from build123d import *

# Parameters (mm, degrees)
SKETCH006_R           = 114.3
PAD003_DEPTH          = 20
SKETCH007_R           = 4.25
HOLE001_DEPTH         = 75
HOLE001_TIPS_R        = 4.25
SKETCH008_R           = 4.25
HOLE002_DEPTH         = 200
POLARPATTERN001_COUNT = 3
POLARPATTERN001_ANGLE = 240


with BuildPart() as part:
    # Sketch006 → Pad003 (new body)
    with BuildSketch(Plane.XY):
        with BuildLine():
            ThreePointArc((50, -124.645457), (0, 134.3), (-50, -124.645457))
            Line((-50, -124.645457), (-50, -154.645457))
            Line((-50, -154.645457), (50, -154.645457))
            Line((50, -154.645457), (50, -124.645457))
        make_face()
        Circle(SKETCH006_R, mode=Mode.SUBTRACT)
    extrude(amount=PAD003_DEPTH)

    # Sketch007 (on Face3 of Pad003) → Hole001 (cut)
    with BuildSketch(Plane.XZ.offset(154.645457)):
        with Locations((-25, 10)):
            Circle(SKETCH007_R)
        with Locations((25, 10)):
            Circle(SKETCH007_R)
    extrude(amount=-HOLE001_DEPTH, mode=Mode.SUBTRACT)

    # Hole001 tips → Hole001 tip 1 section 0
    with BuildSketch(Plane.XZ.offset(79.645457), mode=Mode.PRIVATE) as hole001_tip_1_s0:
        with Locations((-25, 10)):
            Circle(HOLE001_TIPS_R)
    loft([hole001_tip_1_s0.sketch, Vertex(-25, -77.0918, 10)], mode=Mode.SUBTRACT)

    # Hole001 tips → Hole001 tip 2 section 0
    with BuildSketch(Plane.XZ.offset(79.645457), mode=Mode.PRIVATE) as hole001_tip_2_s0:
        with Locations((25, 10)):
            Circle(HOLE001_TIPS_R)
    loft([hole001_tip_2_s0.sketch, Vertex(25, -77.0918, 10)], mode=Mode.SUBTRACT)

    # Sketch008 → Hole002 (cut)
    with BuildSketch(Plane.XZ):
        with Locations((0, 10)):
            Circle(SKETCH008_R)
    hole002 = extrude(amount=-HOLE002_DEPTH, mode=Mode.SUBTRACT)

    # PolarPattern001: Hole002 ×3 about axis
    polarpattern001_axis = Axis((0, 0, 0), (0, 0, 1))
    for i in range(1, POLARPATTERN001_COUNT):
        add(hole002.rotate(polarpattern001_axis, i * POLARPATTERN001_ANGLE / (POLARPATTERN001_COUNT - 1)), mode=Mode.SUBTRACT)


solid = part.part
Input: part model. Units: mm. Frame: model coordinates. A direction names the side the tool comes from. Give positions to 0.01 mm unless a question says otherwise; leave off trailing zeros. Order: outer loops, then holes, each group sorted by start corner. A loop starts at its lowest first (then second) coordinate and runs counter-clockwise, first axis right, second up. Notation, with made-up numbers: (30.25, 75.5) - (84.25, 75.5) arc R38 ccw to (84.25, 113.5) - close; hole circle Ø2 at (74, 42.25). An arc over 180 degrees is marked (long way). Answer as a JSON object with one key per item and string values. Group by question number.
Q1. First-contact query: pin 1 Ø1.5 at (y, z) = (-45.5, 16.5) entering from +X; pin 2 Ø3 at (x, z) = (22.5, 11) entering from +Y; pin 3 Ø10 at (y, z) = (-108, 5) entering from +X; pin 4 Ø8 at (x, y) = (-62, 102) entering from -Z. Flat tips, straight axial feed; report the tip coordinate or a pass-through.
Q2. Cut plane C-C, the plane x = -72.5. Output: boundary loops of the cut face in (y, z), then the cut area to 3 significant figures.
Q3. Mould query, pull axis Y, two halves, no side actions, for faces 1 (the face through (-14.88, 113.327, 9.86)), 2 (the face through (5.2, 134.2, 9.9)), 3 (the face through (-109.52, -58.55, 11.28)), 4 (the face through (-1, -117, 20)). Classes: pulls with the +Y half, pulls with the -Y half, needs draft (parallel to the pull), parting line crosses it, or undercut.
Q4. Cut plane D-D, the plane z = 10. Output: boundary loops of the cut face in (x, y).
Q5. Cut plane B-B, the plane x = 0. Output: boundary loops of the cut face in (y, z), then the cut area to 3 significant figures.
Q6. Set-up query: faces 5 (the face through (24.08, -132.88, 5.85)), 6 (the face through (-0.92, 124.12, 5.85)), 7 (the face through (-50, -139, 10)). Return all of +Z, -Z, +X, -X, +Y, -Y with unobstructed straight access to the full face (end or side cutting, diameter ignored); none if empty.
Q7. Line query: probe 1 along X at (y, z) = (-129, 10); probe 2 along Z at (x, y) = (0, 123.5); probe 3 along X at (y, z) = (43, 14). Output: solid intervals per line, ascending.
Q8. Cut plane A-A, the plane y = 0. Output: boundary loops of the cut face in (x, z), then the cut area to 3 significant figures.
Results:
{
 "1": {"pin 1": "x = 126.63", "pin 2": "y = 132.65", "pin 3": "x = 86.18", "pin 4": "z = 0"},
 "2": {"outline": "(-113.05, 0) - (-88.36, 0) - (-88.36, 20) - (-113.05, 20) - close; (88.36, 0) - (113.05, 0) - (113.05, 20) - (88.36, 20) - close", "area": "987 mm^2"},
 "3": {"face 1": "undercut", "face 2": "parting line crosses it", "face 3": "undercut", "face 4": "needs draft"},
 "4": {"outline": "(-118.37, -63.44) - (-101.04, -53.43) arc R114.3 cw to (-4.25, 114.22) - (-4.25, 134.23) arc R134.3 ccw to start; (-114.12, -70.8) arc R134.3 ccw to (-50, -124.65) - (-50, -154.65) - (-29.25, -154.65) - (-29.25, -110.49) arc R114.3 cw to (-96.79, -60.79) - close; (-20.75, -154.65) - (20.75, -154.65) - (20.75, -112.4) arc R114.3 cw to (-20.75, -112.4) - close; (4.25, 114.22) arc R114.3 cw to (101.04, -53.43) - (118.37, -63.44) arc R134.3 ccw to (4.25, 134.23) - close; (29.25, -154.65) - (50, -154.65) - (50, -124.65) arc R134.3 ccw to (114.12, -70.8) - (96.79, -60.79) arc R114.3 cw to (29.25, -110.49) - close"},
 "5": {"outline": "(-154.65, 0) - (-114.3, 0) - (-114.3, 20) - (-154.65, 20) - close; (114.3, 0) - (134.3, 0) - (134.3, 5.75) - (114.3, 5.75) - close; (114.3, 14.25) - (134.3, 14.25) - (134.3, 20) - (114.3, 20) - close", "area": "1,040 mm^2"},
 "6": {"face 5": "-Y", "face 6": "+Y", "face 7": "+Z, -Z, -X, -Y"},
 "7": {"probe 1": "-50 to -29.25, -20.75 to 20.75, 29.25 to 50", "probe 2": "0 to 5.75, 14.25 to 20", "probe 3": "-127.23 to -105.9, 105.9 to 127.23"},
 "8": {"outline": "(-134.3, 0) - (-114.3, 0) - (-114.3, 20) - (-134.3, 20) - close; (114.3, 0) - (134.3, 0) - (134.3, 20) - (114.3, 20) - close", "area": "800 mm^2"}
}
